from build123d import *

# Parameters (mm, degrees)
F0_R          = 10
F0_R_2        = 5
F1_DEPTH      = 20
F2_W          = 15
F2_H          = 20
F3_DEPTH      = 20
F4_R          = 5
F5_DEPTH      = 20.001
F6_W          = 10
F6_H          = 5
F7_DEPTH      = 10.001
F7_DEPTH_BACK = 20.001


with BuildPart() as f1:
    # F0 (on Front) → F1 (new body)
    with BuildSketch(Plane.XZ):
        Circle(F0_R)
        Circle(F0_R_2, mode=Mode.SUBTRACT)
    extrude(amount=-F1_DEPTH)

    # F2 (on Right) → F3 (join)
    with BuildSketch(Plane.YZ):
        with Locations((12.5, 0.2303563431)):
            Rectangle(F2_W, F2_H)
    extrude(amount=F3_DEPTH)

    # F4 (on Front) → F5 (cut, through all)
    with BuildSketch(Plane.XZ):
        Circle(F4_R)
    extrude(amount=-F5_DEPTH, mode=Mode.SUBTRACT)

    # F6 (on Right) → F7 (cut, two sides)
    with BuildSketch(Plane.YZ) as f7_sk:
        with Locations((5, -0.1396772545)):
            Rectangle(F6_W, F6_H)
    extrude(amount=-F7_DEPTH, mode=Mode.SUBTRACT)
    extrude(f7_sk.sketch, amount=F7_DEPTH_BACK, mode=Mode.SUBTRACT)


solid = f1.part
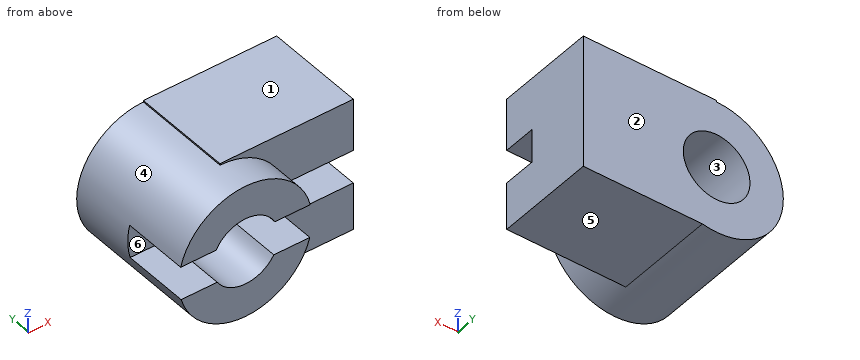
Work out the finished part from the listing and answer in its coordinate system (mm). Face numbers are marked on the shaded views. A direction names the side the tool comes from. Coordinates: 2 decimals unless noted, no trailing zeros. Order: outer loops, then holes, each group sorted by start corner. A loop starts at its lowest first (then second) coordinate and runs counter-clockwise, first axis right, second up. Notation, with made-up numbers: (51, 2.25) - (65, 2.25) arc R33 ccw to (65, 39.25) - close; hole circle Ø4 at (60, -37.5). An arc over 180 degrees is marked (long way). Put each result on its own line as item: value. Start each with the question number.
1) Find section B-B (y = 8.5). Give the vertices of the cut face in (x, z).
2) Flat-ended cylindrical pins translate along their axes: pin 1 (3.5 mm diameter, centred on x = 10.5, z = -7, fed in from -Y); pin 2 (8 mm diameter, centred on x = 11, y = 6.5, fed in from -Z); pin 3 (2 mm diameter, centred on y = 17.5, z = 1.5, fed in from -X). Find the tip coordinate at first contact, or state that the pin passes through.
3) Find section C-C (x = -1.5). Give the vertices of the cut face in (y, z).
4) For the marked faces 4, 5 and 6, determine the directions among +Z, -Z, +X, -X, +Y, -Y from which every point of the face is accessible in a straight line to the end or side of a thin tool.
5) Find section A-A (z = 0). Give the vertices of the cut face in (x, y), plus the area to 3 significant figures.
6) For a pull along Z with two mould halves and no side action, classify the marked faces 1, 2 and 3 as released by +Z, released by -Z, zero draft, split by the parting line, or undercut.
7) Find the intervals of material crossed by line 1 (Z direction, x = 16.75, y = 8.75); line 2 (Z direction, x = 0.25, y = 7.5); line 3 (X direction, y = 2.25, z = 2.5), in increasing order. Write a range as from..to.
8) Find section D-D (x = 6). Give the vertices of the cut face in (y, z), plus the area to 3 significant figures.
Results list:
1. outline: (-9.72, 2.36) - (-4.41, 2.36) arc R5 cw to (4.41, 2.36) - (20, 2.36) - (20, 10.23) - (0, 10.23) - (0, 10) arc R10 ccw to start; (-9.65, -2.64) arc R10 ccw to (2.13, -9.77) - (20, -9.77) - (20, -2.64) - (4.25, -2.64) arc R5 cw to (-4.25, -2.64) - close
2. pin 1: stops at y = 5
2. pin 2: stops at z = -9.77
2. pin 3: stops at x = -9.99
3. outline: (0, -9.89) - (20, -9.89) - (20, -4.77) - (0, -4.77) - close; (0, 4.77) - (20, 4.77) - (20, 9.89) - (0, 9.89) - close
4. face 4: -Y
4. face 5: -Z, +X, +Y, -Y
4. face 6: +X, -X, -Y
5. outline: (-10, 10) - (-5, 10) - (-5, 20) - (-10, 20) - close; (5, 10) - (20, 10) - (20, 20) - (5, 20) - close
5. area: 200 mm^2
6. face 1: released by +Z
6. face 2: zero draft
6. face 3: undercut
7. line 1: z = -9.77..-2.64, 2.36..10.23
7. line 2: z = -10..-4.99, 4.99..10.23
7. line 3: x = -9.68..-4.33, 4.33..9.68
8. outline: (0, -8) - (5, -8) - (5, -9.77) - (20, -9.77) - (20, 10.23) - (5, 10.23) - (5, 8) - (0, 8) - (0, 2.36) - (10, 2.36) - (10, -2.64) - (0, -2.64) - close
8. area: 330 mm^2
